Design review of the part built by this model. Coordinates are the model's own, in mm. A direction names the side the tool comes from. Coordinates: 2 decimals unless noted, no trailing zeros. Loops run counter-clockwise (first coordinate to the right, second up) from the corner with the lowest first, then second, coordinate; pieces in that order, holes last. Notation, with made-up numbers: (-33, 80.25) -> (11, 80.25) arc R28 cw to (11, 114.25) -> close; hole circle Ø7 at (72.5, -4). An arc over 180 degrees is marked (long way). Answer as a JSON object with one key per item and string values.
Autodesk Inventor part; units mm, degrees
ref_plane "YZ Plane" through (0, 0, 0) normal (1, 0, 0) x (0, 1, 0)
ref_plane "XZ Plane" through (0, 0, 0) normal (0, 1, 0) x (-1, 0, 0)
ref_plane "XY Plane" through (0, 0, 0) normal (0, 0, 1) x (1, 0, 0)
sketch "Sketch2" plane through (0, 0, 0) normal (0, 0, 1) x (1, 0, 0)
  line L0 (0, 0) -> (0, 20) construction
  line L1 (0, 20) -> (0, 40) construction
  line L2 (0, 0) -> (20, 0) construction
  line L3 (20, 0) -> (40, 0) construction
  line L4 (-10, -10) -> (-10, 50)
  line L5 (-10, 50) -> (10, 50)
  line L6 (10, 50) -> (10, 30)
  line L7 (10, 30) -> (30, 10)
  line L8 (30, 10) -> (50, 10)
  line L9 (50, 10) -> (50, -10)
  line L10 (50, -10) -> (-10, -10)
  dimension "d0" = 20
  dimension "d1" = 20
  dimension "d2" = 60
  dimension "d3" = 10
  dimension "d4" = 10
  dimension "d5" = 10
extrude "Extrusion1" add sketch "Sketch2" along normal blind 5
hole "Hole1" at (0, 40, 0) at (0, 20, 0) at (20, 0, 0) at (40, 0, 0) at (0, 0, 0) direction (0, 0, 1) diameter 5.5 end through all
fillet "Fillet1" radius 2 7 edges at (-10, 50, 2.5) (10, 50, 2.5) (10, 30, 2.5) (-10, -10, 2.5) (30, 10, 2.5) (50, 10, 2.5) (50, -10, 2.5)
properties part number "6060L"
1) For faces 1 (the flat face through (39, 10, 2)), 2 (the flat face through (50, 0, 2)), list the 3-axis set-ups (+Z, -Z, +X, -X, +Y, -Y) from which the entire face can be reached by the end or side of a thin tool; tool diameter is ignored.
Completed:
{"face 1": "+Z, -Z, +X, +Y", "face 2": "+Z, -Z, +X, +Y, -Y"}
2) Wall thickness on probe 1 along X at (y, z) = (0, 2.8); probe 2 along Y at (x, z) = (1, 2.45): over which ranges is each line inside the solid? List them lowest first.
Completed:
{"probe 1": "-10 to -2.75, 2.75 to 17.25, 22.75 to 37.25, 42.75 to 50", "probe 2": "-10 to -2.56, 2.56 to 17.44, 22.56 to 37.44, 42.56 to 50"}
3) Clearance check with flat-ended pins moving along their axes: pin 1 Ø2 at (y, z) = (28.5, 4.5) entering from +X; pin 2 Ø3 at (x, z) = (36.5, 4) entering from +Y; pin 3 Ø2 at (y, z) = (29.5, 3.5) entering from +X; pin 4 Ø6.5 at (x, y) = (0, 0) entering from +Z. State where each tip first meets the part, or that it passes through.
Completed:
{"pin 1": "x = 12.5", "pin 2": "y = 10", "pin 3": "x = 11.5", "pin 4": "z = 5"}
4) Add section B-B, the plane y = 40. Give the boundary of the cut face in (x, z).
Completed:
{"outline": "(-10, 0) -> (-2.75, 0) -> (-2.75, 5) -> (-10, 5) -> close; (2.75, 0) -> (10, 0) -> (10, 5) -> (2.75, 5) -> close"}
5) Add section D-D, the plane y = -1. Give the boundary of the cut face in (x, z).
Completed:
{"outline": "(-10, 0) -> (-2.56, 0) -> (-2.56, 5) -> (-10, 5) -> close; (2.56, 0) -> (17.44, 0) -> (17.44, 5) -> (2.56, 5) -> close; (22.56, 0) -> (37.44, 0) -> (37.44, 5) -> (22.56, 5) -> close; (42.56, 0) -> (50, 0) -> (50, 5) -> (42.56, 5) -> close"}
6) Add section A-A, the plane x = 20. Give the boundary of the cut face in (y, z).
Completed:
{"outline": "(-10, 0) -> (-2.75, 0) -> (-2.75, 5) -> (-10, 5) -> close; (2.75, 0) -> (20, 0) -> (20, 5) -> (2.75, 5) -> close"}
7) Add section C-C, the plane z = 3.4. Give the boundary of the cut face in (x, y).
Completed:
{"outline": "(-10, -8) arc R2 ccw to (-8, -10) -> (48, -10) arc R2 ccw to (50, -8) -> (50, 8) arc R2 ccw to (48, 10) -> (30.83, 10) arc R2 cw to (29.41, 10.59) -> (10.59, 29.41) arc R2 cw to (10, 30.83) -> (10, 48) arc R2 ccw to (8, 50) -> (-8, 50) arc R2 ccw to (-10, 48) -> close; hole circle Ø5.5 at (0, 0); hole circle Ø5.5 at (0, 20); hole circle Ø5.5 at (0, 40); hole circle Ø5.5 at (20, 0); hole circle Ø5.5 at (40, 0)"}
8) The part is to be moulded in two halves that separate along Y. For faces 3 (the cylindrical face through (17.273, -0.358, 2.535)), 4 (the flat face through (10, 40, 2)), 5 (the flat face through (0, 50, 2)), 6 (the cylindrical face through (-0.121, 17.253, 2.535)), say which applies: pulls with the +Y half, pulls with the -Y half, needs draft (parallel to the pull), parting line crosses it, or undercut.
Completed:
{"face 3": "undercut", "face 4": "needs draft", "face 5": "pulls with the +Y half", "face 6": "undercut"}
